```python
from build123d import *

# Parameters (mm, degrees)
SKETCH1_W                  = 698.5
SKETCH1_H                  = 327.152
BOSS_EXTRUDE1_DEPTH        = 3.175
F_9_0_196_DIAMETER_HOLE2_D = 4.9784


with BuildPart() as part:
    # Sketch1 → Boss-Extrude1 (new body)
    with BuildSketch(Plane(origin=(0, 0, 0), x_dir=(0, 1, 0), z_dir=(0, 0, 1))):
        Rectangle(SKETCH1_W, SKETCH1_H)
    extrude(amount=BOSS_EXTRUDE1_DEPTH)

    # #9 (0.196) Diameter Hole2 (through all)
    with Locations(Plane.XY.offset(3.175)):
        with Locations((-150.876, 336.55), (-125.476, 336.55), (65.024, 336.55), (90.424, 336.55), (90.424, -336.55), (65.024, -336.55), (-125.476, -336.55), (-150.876, -336.55), (-371.836153613, -199.719855434), (150.876, 133.35), (150.876, 107.95), (150.876, -107.95), (150.876, -133.35)):
            Hole(F_9_0_196_DIAMETER_HOLE2_D / 2)


solid = part.part
```
The model under review builds one solid part; all positions refer to its coordinate system, in mm. Round coordinates to 2 decimals unless told otherwise and drop trailing zeros. Use one line per item in the form item = value.
Q1. Draft analysis for pull direction Z (two halves, no side actions). For faces 1 (the flat face through (-2, -5, 3.175)), 2 (the flat face through (-2, -5, 0)), state which applies: +Z half, -Z half, draft (parallel to the pull), parting line (faces both ways), or undercut.
Answer key:
face_1 = +Z half
face_2 = -Z half
Q2. For line 1 (X direction, y = -336.55, z = 1.55); line 2 (Y direction, x = 150.5, z = 1.9), list the stretches that pass through material, from the lowest coordinate up. Write a range as [from, to].
Answer key:
line_1 = [-163.58, -153.37], [-148.39, -127.97], [-122.99, 62.53], [67.51, 87.93], [92.91, 163.58]
line_2 = [-349.25, -135.81], [-130.89, -110.41], [-105.49, 105.49], [110.41, 130.89], [135.81, 349.25]
Q3. Insertion check: pin 1 Ø4.5 at (x, y) = (150.876, -107.95) entering from +Z. The pin has a flat end and moves straight along its axis. Give the tip position at first contact, or say it passes through.
Answer key:
pin_1 = through
